from build123d import *

# Parameters (mm, degrees)
SKETCH_1_R               = 6
EXTRUDE_1_DEPTH          = 80
SKETCH_2_R               = 4.5
EXTRUDE_2_DEPTH          = 10
EXTRUDE_START            = 5
SKETCH_3_R               = 6
EXTRUDE_3_DEPTH          = 5
CUT_EXTRUDE_1_DEPTH      = 81.448741444
CUT_EXTRUDE_1_DEPTH_BACK = 81.448741444
SKETCH_4_R               = 1.5


with BuildPart() as part:
    # Эскиз1 → Бобышка-Вытянуть1 (new body)
    with BuildSketch(Plane(origin=(0, 0, 0), x_dir=(1, 0, 0), z_dir=(0, 1, 0))):
        with Locations(Location((0, 0, 0), (0, 0, 270))):
            Circle(SKETCH_1_R)
    extrude(amount=-EXTRUDE_1_DEPTH)

    # Эскиз2 → Бобышка-Вытянуть2 (add)
    with BuildSketch(Plane(origin=(0, 0, 0), x_dir=(1, 0, 0), z_dir=(0, 1, 0))):
        with Locations(Location((0, 0, 0), (0, 0, 270))):
            Circle(SKETCH_2_R)
    extrude(amount=EXTRUDE_2_DEPTH)

    # Эскиз3 → Бобышка-Вытянуть3 (add)
    with BuildSketch(Plane(origin=(0, 0, 0), x_dir=(1, 0, 0), z_dir=(0, 1, 0)).offset(EXTRUDE_START)):
        with Locations(Location((0, 0, 0), (0, 0, 270))):
            Circle(SKETCH_3_R)
    extrude(amount=-EXTRUDE_3_DEPTH)

    # Эскиз4 → Вырез-Вытянуть1 (cut, two sides: drawn at the far end of the back side and taken through both)
    with BuildSketch(Plane(origin=(0, 0, 0), x_dir=(0, 0, -1), z_dir=(1, 0, 0)).offset(-CUT_EXTRUDE_1_DEPTH_BACK)):
        with Locations((0, 2.5)):
            Circle(SKETCH_4_R)
    extrude(amount=CUT_EXTRUDE_1_DEPTH + CUT_EXTRUDE_1_DEPTH_BACK, mode=Mode.SUBTRACT)


solid = part.part
Check sheet for the modelled part. Datum: model origin and axes. Units: mm. A direction names the side the tool comes from. Give positions to 0.01 mm unless a question says otherwise; leave off trailing zeros. Write each loop counter-clockwise with the first axis right and the second up, starting at its lowest first coordinate (ties: lowest second). Pieces come first, ordered by that corner, then holes. Notation, with made-up numbers: M 67,-34 L 73,-34 A9 cw 73,-28 Z; hole C 88,63.25 d11. An arc over 180 degrees is marked long. Use one line per item in the form item = value.
(1) Draft check along Z on faces 1 (the cylindrical face through (0, 1, 0)), 2 (the cylindrical face through (1.352, 7.465, 4.292)), 3 (the flat face through (0, -80, 0)). Enter one of: pulls with the +Z half, pulls with the -Z half, needs draft (parallel to the pull), parting line crosses it, or undercut.
Answer block:
face_1 = undercut
face_2 = parting line crosses it
face_3 = needs draft
(2) Tool access check on faces 4 (the flat face through (4.5, 5, -1.4)), 5 (the cylindrical face through (1.802, -36.905, 5.723)). Record the directions out of +Z, -Z, +X, -X, +Y, -Y that give a thin tool (end or side, any length) a straight path to the whole face; none if there is none.
Answer block:
face_4 = +Y
face_5 = +Y, -Y
(3) Section check B-B on x = 0. Record the boundary of the cut face in (y, z).
Answer block:
outline = M -80,-6 L 5,-6 L 5,-4.5 L 10,-4.5 L 10,4.5 L 5,4.5 L 5,6 L -80,6 Z; hole C 2.5,0 d3
(4) Section check A-A on z = 0. Record the boundary of the cut face in (x, y).
Answer block:
outline = M -6,-80 L 6,-80 L 6,1 L -6,1 Z; M -6,4 L 6,4 L 6,5 L 4.5,5 L 4.5,10 L -4.5,10 L -4.5,5 L -6,5 Z
(5) Material ranges on line 1 along Y through (x, z) = (-2.75, -1.25); line 2 along Y through (x, z) = (2, 0); line 3 along Z through (x, y) = (3, 2.5), recorded low to high.
Answer block:
line_1 = -80 to 1.67, 3.33 to 10
line_2 = -80 to 1, 4 to 10
line_3 = -5.2 to -1.5, 1.5 to 5.2
(6) Depth check by flat-ended pin: P1, Ø5, axis at y = -35.5, z = -3, coming from the +X side; P2, Ø6, axis at x = -3.5, y = -64, coming from the -Z side; P3, Ø6, axis at y = -55.5, z = -2.5, coming from the -X side. Enter the tip coordinate at first touch or a pass-through.
Answer block:
P1 = 5.98
P2 = -5.98
P3 = -6
(7) Section check C-C on z = 3.5. Record the boundary of the cut face in (x, y), plus the area to 3 significant figures.
Answer block:
outline = M -4.87,-80 L 4.87,-80 L 4.87,5 L 2.83,5 L 2.83,10 L -2.83,10 L -2.83,5 L -4.87,5 Z
area = 857 mm2
(8) Section check D-D on y = 2.5. Record the boundary of the cut face in (x, z), plus the area to 3 significant figures.
Answer block:
outline = M -5.81,-1.5 A6 ccw 5.81,-1.5 Z; M -5.81,1.5 L 5.81,1.5 A6 ccw Z
area = 77.5 mm2
